```python
from build123d import *

# Parameters (mm, degrees)
F0_W     = 78.157008
F0_H     = 51.731035
F1_DEPTH = 63.5
F3_DEPTH = 51.732035
F4_W     = 50.8
F4_H     = 38.1
F5_DEPTH = 50.8


with BuildPart() as f1:
    # F0 (on Front) → F1 (new body)
    with BuildSketch(Plane.XZ):
        with Locations((39.078504, 25.865517)):
            Rectangle(F0_W, F0_H)
    extrude(amount=-F1_DEPTH)

    # F2 (on face) → F3 (cut, through all)
    with BuildSketch(Plane.XY.offset(51.731035)):
        Polygon((78.157008, 25.4), (0, 0), (78.157008, 0), align=None)
    extrude(amount=-F3_DEPTH, mode=Mode.SUBTRACT)

    # F4 (on Front) → F5 (cut)
    with BuildSketch(Plane.XZ):
        with Locations((52.757008, 32.681035)):
            Rectangle(F4_W, F4_H)
    extrude(amount=-F5_DEPTH, mode=Mode.SUBTRACT)


solid = f1.part
```
Work out the finished part from the listing and answer in its coordinate system (mm). A direction names the side the tool comes from. Give positions to 0.01 mm unless a question says otherwise; leave off trailing zeros. Loops run counter-clockwise (first coordinate to the right, second up) from the corner with the lowest first, then second, coordinate; pieces in that order, holes last. Notation, with made-up numbers: (67.25, 28.25) -> (71.25, 28.25) arc R19 ccw to (71.25, 37.25) -> close; hole circle Ø1 at (83, 7.25). An arc over 180 degrees is marked (long way). One line per question, with ' | ' between items. Start each with the question number.
1) For faces 1 (the face through (52, 34, 13.631)), 2 (the face through (21, 38, 51.731)), determine the directions among +Z, -Z, +X, -X, +Y, -Y from which every point of the face is accessible in a straight line to the end or side of a thin tool.
2) Section C-C, the plane x = 47 is taken. Determine the outline of the cut face in (y, z), then the cut area to 3 significant figures.
3) Each of these flat-tipped pins is pushed along its axis until it touches: pin 1 (2 mm diameter, centred on y = 57, z = 42.5, fed in from -X); pin 2 (6 mm diameter, centred on x = 54.5, z = 43, fed in from -Y); pin 3 (8 mm diameter, centred on x = 17, z = 34.5, fed in from -Y); pin 4 (8 mm diameter, centred on x = 47, z = 17.5, fed in from -Y). Where does it stop, or does it pass through?
4) Straight lines are drawn through the part: L1, parallel to Y at x = 55, z = 21; L2, parallel to Z at x = 71, y = 33; L3, parallel to X at y = 47, z = 22. For each, find the intervals that lie inside material, in ascending order.
5) Section B-B, the plane z = 7 is taken. Determine the outline of the cut face in (x, y).
6) Section D-D, the plane y = 5.5 is taken. Determine the outline of the cut face in (x, z), then the cut area to 3 significant figures.
7) Determine the mould class of faces 3 (the face through (0, 31, 26)), 4 (the face through (27.357, 30, 32)), 5 (the face through (39, 38, 0)) for opening direction X: +X half, -X half, draft (parallel to the pull), parting line (faces both ways), or undercut.
8) Section A-A, the plane y = 33.5 is taken. Determine the outline of the cut face in (x, z), then the cut area to 3 significant figures.
Resolved:
1) face 1: +Z, +X, -Y | face 2: +Z, +X, -X, +Y, -Y
2) outline: (15.27, 0) -> (63.5, 0) -> (63.5, 51.73) -> (50.8, 51.73) -> (50.8, 13.63) -> (15.27, 13.63) -> close | area: 1,140 mm2
3) pin 1: x = 0 | pin 2: y = 50.8 | pin 3: y = 4.22 | pin 4: y = 14.94
4) L1: 50.8 to 63.5 | L2: 0 to 13.63 | L3: 0 to 27.36
5) outline: (0, 0) -> (78.16, 25.4) -> (78.16, 63.5) -> (0, 63.5) -> close
6) outline: (0, 0) -> (16.92, 0) -> (16.92, 51.73) -> (0, 51.73) -> close | area: 875 mm2
7) face 3: -X half | face 4: +X half | face 5: draft
8) outline: (0, 0) -> (78.16, 0) -> (78.16, 13.63) -> (27.36, 13.63) -> (27.36, 51.73) -> (0, 51.73) -> close | area: 2,110 mm2
